from build123d import *

# Parameters (mm, degrees)
SKETCH1_W           = 1.5875
SKETCH1_H           = 155.8925
BOSS_EXTRUDE1_DEPTH = 381
CUT_EXTRUDE1_DEPTH  = 1.5875
FILLET1_R           = 6.35


with BuildPart() as part:
    # Sketch1 → Boss-Extrude1 (new body)
    with BuildSketch(Plane(origin=(0, 0, 0), x_dir=(1, 0, 0), z_dir=(0, 1, 0))):
        with Locations((0.79375, 77.94625)):
            Rectangle(SKETCH1_W, SKETCH1_H)
    extrude(amount=BOSS_EXTRUDE1_DEPTH)

    # Sketch2 → Cut-Extrude1 (cut)
    with BuildSketch(Plane.ZY):
        Polygon((-39.0525, 381), (-155.8925, 214.122), (-155.8925, 381), align=None)
    extrude(amount=-CUT_EXTRUDE1_DEPTH, mode=Mode.SUBTRACT)

    # Fillet1
    fillet1_edges = [part.edges().sort_by_distance(p)[0] for p in [
        (0.79375, 381, -39.0525),
        (0.79375, 214.122, -155.8925),
        (0.79375, 381, 0),
        (0.79375, 0, -155.8925),
        (0.79375, 0, 0),
    ]]
    fillet(fillet1_edges, radius=FILLET1_R)


solid = part.part
Verification items for the finished model (mm, model axes). Give positions to 0.01 mm unless a question says otherwise; leave off trailing zeros. Loops run counter-clockwise (first coordinate to the right, second up) from the corner with the lowest first, then second, coordinate; pieces in that order, holes last.
1) Sectioned sample at A-A, the plane x = 0.9. Enter the section's corners in (y, z), then the cut area to 3 significant figures.
2) Thickness scan on line 1 along Y through (x, z) = (0.5, -41); line 2 along Y through (x, z) = (1, -76.5); line 3 along Z through (x, y) = (0.9, 312.5). Record the ranges inside material, lowest first.
3) Sectioned sample at B-B, the plane z = -54.5. Enter the section's corners in (x, y), then the cut area to 3 significant figures.
4) Sectioned sample at C-C, the plane y = 350. Enter the section's corners in (x, z), then the cut area to 3 significant figures.
Answers:
1. outline: (0, -149.54) arc R6.35 ccw to (6.35, -155.89) - (212.12, -155.89) arc R6.35 ccw to (215.76, -154.74) - (378.29, -40.95) arc R6.35 ccw to (381, -35.75) - (381, -6.35) arc R6.35 ccw to (374.65, 0) - (6.35, 0) arc R6.35 ccw to (0, -6.35) - close
1. area: 49,600 mm2
2. line 1: y = 0 to 378.22
2. line 2: y = 0 to 327.52
2. line 3: z = -87.01 to 0
3. outline: (0, 0) - (1.59, 0) - (1.59, 358.94) - (0, 358.94) - close
3. area: 570 mm2
4. outline: (0, -60.76) - (1.59, -60.76) - (1.59, 0) - (0, 0) - close
4. area: 96.5 mm2
